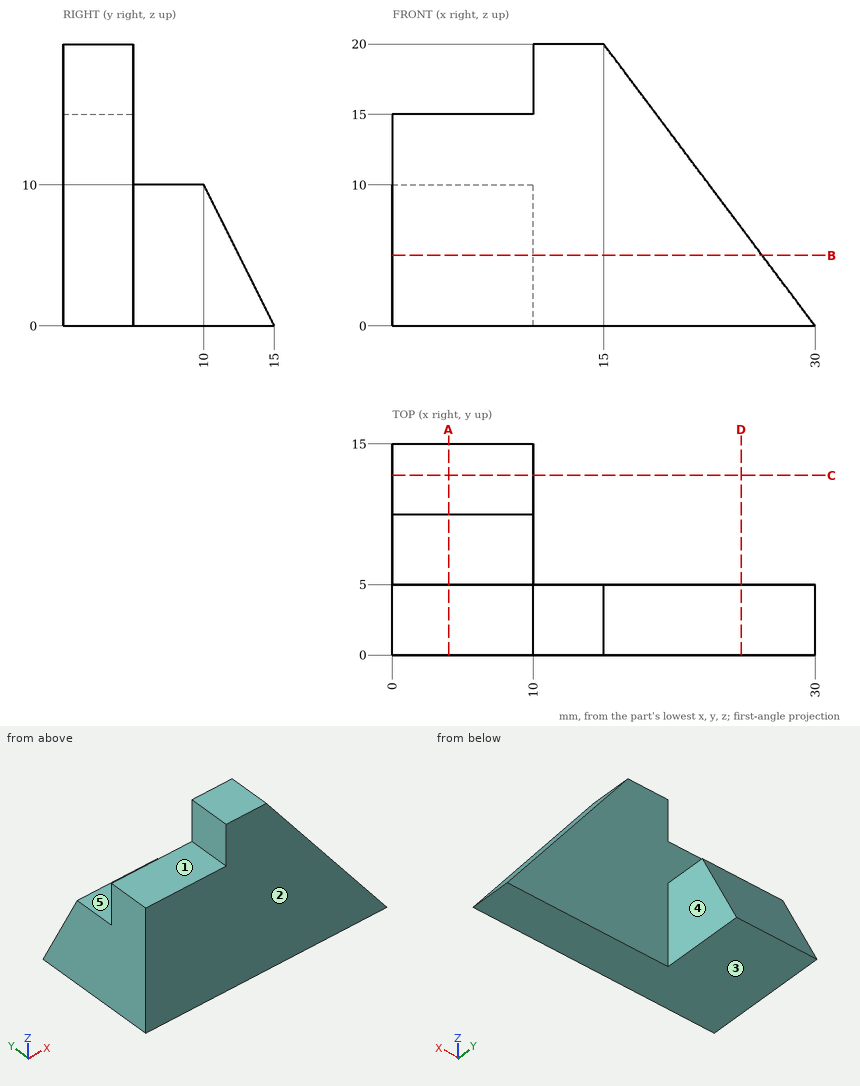
Could you check a few things on this drawing? It's one solid part, dimensions in mm from its lowest x, y, z. A direction names the side the tool comes from. Coordinates: 2 decimals unless noted, no trailing zeros. Write each loop counter-clockwise with the first axis right and the second up, starting at its lowest first coordinate (ties: lowest second). Pieces come first, ordered by that corner, then holes. Notation, with made-up numbers: M 43,22 L 84,22 A25 ccw 84,60 Z; hole C 56,5 d11. An arc over 180 degrees is marked long. Answer as CSV lines item,"result". Start each with the question number.
Q1. Will these pins go through, and if not, where does the flat tip stop? pin 1 Ø1.5 at (x, z) = (13, 13.5) entering from -Y; pin 2 Ø2 at (x, y) = (3, 13) entering from +Z; pin 3 Ø2.5 at (x, y) = (4.5, 7) entering from +Z; pin 4 Ø8 at (x, z) = (6.5, 8.5) entering from +Y.
Q2. Suppose I cut it at B-B, the plane z = 5. List the corners of the cut face in (x, y) for me.
Q3. I need wall thicknesses on probe 1 along Z at (x, y) = (7.75, 1); probe 2 along Y at (x, z) = (13.75, 13.75); probe 3 along Z at (x, y) = (5, 6). Which ranges of each line are inside material? Lowest first, please. Write a range as [from, to].
Q4. Suppose I cut it at C-C, the plane y = 12.75. List the corners of the cut face in (x, z) for me, then the cut area to 3 significant figures.
Q5. For the marked faces 1, 2, 3, 4 and 5, which set-ups out of +Z, -Z, +X, -X, +Y, -Y let a thin tool reach every point of the face, with its end or its side?
Q6. Suppose I cut it at D-D, the plane x = 24.75. List the corners of the cut face in (y, z) for me, then the cut area to 3 significant figures.
Q7. Suppose I cut it at A-A, the plane x = 4. List the corners of the cut face in (y, z) for me, then the cut area to 3 significant figures.
Entries:
1,pin 1,"stops at y = 0"
1,pin 2,"stops at z = 6"
1,pin 3,"stops at z = 10"
1,pin 4,"stops at y = 12.75"
2,outline,"M 0,0 L 26.25,0 L 26.25,5 L 10,5 L 10,12.5 L 0,12.5 Z"
3,probe 1,"z = [0, 15]"
3,probe 2,"y = [0, 5]"
3,probe 3,"z = [0, 10]"
4,outline,"M 0,0 L 10,0 L 10,4.5 L 0,4.5 Z"
4,area,"45.0 mm²"
5,face 1,"+Z, -X, +Y, -Y"
5,face 2,"+Z, -Z, +X, -X, -Y"
5,face 3,"-Z, +X, -X, +Y, -Y"
5,face 4,"+Z, -Z, +X, +Y"
5,face 5,"+Z, +X, -X, +Y"
6,outline,"M 0,0 L 5,0 L 5,7 L 0,7 Z"
6,area,"35.0 mm²"
7,outline,"M 0,0 L 15,0 L 10,10 L 5,10 L 5,15 L 0,15 Z"
7,area,"150 mm²"
